```python
from build123d import *

# Parameters (mm, degrees)
F0_R     = 63.5
F1_DEPTH = 3.175


with BuildPart() as f1:
    # F0 (on Right) → F1 (new body)
    with BuildSketch(Plane.YZ):
        Circle(F0_R)
        with BuildLine():
            ThreePointArc((42.207203769, 42.207203769), (55.1463692956, 22.8423740779), (59.69, 0))
            ThreePointArc((59.69, 0), (56.4919386946, -19.2758128889), (47.240445216, -36.486112917))
            ThreePointArc((47.240445216, -36.486112917), (44.8152116738, -39.4270580012), (42.207203769, -42.207203769))
            ThreePointArc((42.207203769, -42.207203769), (22.8423740779, -55.1463692956), (0, -59.69))
            ThreePointArc((0, -59.69), (-19.2758128889, -56.4919386946), (-36.486112917, -47.240445216))
            ThreePointArc((-36.486112917, -47.240445216), (-39.4270580012, -44.8152116738), (-42.207203769, -42.207203769))
            ThreePointArc((-42.207203769, -42.207203769), (-55.1463692956, -22.8423740779), (-59.69, 0))
            ThreePointArc((-59.69, 0), (-56.4919386946, 19.2758128889), (-47.240445216, 36.486112917))
            ThreePointArc((-47.240445216, 36.486112917), (-44.8152116738, 39.4270580012), (-42.207203769, 42.207203769))
            ThreePointArc((-42.207203769, 42.207203769), (-22.8423740779, 55.1463692956), (0, 59.69))
            ThreePointArc((0, 59.69), (19.2758128889, 56.4919386946), (36.486112917, 47.240445216))
            ThreePointArc((36.486112917, 47.240445216), (39.4270580012, 44.8152116738), (42.207203769, 42.207203769))
        make_face(mode=Mode.SUBTRACT)
        with BuildLine():
            ThreePointArc((29.845, -29.845), (16.7276475457, -19.8525445451), (6.7351920908, -6.7351920908))
            ThreePointArc((6.7351920908, -6.7351920908), (3.6450596933, -8.7999525472), (0, -9.525))
            ThreePointArc((0, -9.525), (8.5432084009, -25.5734757664), (22.6607951031, -37.0292048969))
            Line((22.6607951031, -37.0292048969), (29.845, -29.845))
        make_face()
        with BuildLine():
            ThreePointArc((-6.7351920908, 6.7351920908), (-3.6450596933, 8.7999525472), (0, 9.525))
            ThreePointArc((0, 9.525), (-8.5432084009, 25.5734757664), (-22.6607951031, 37.0292048969))
            Line((-22.6607951031, 37.0292048969), (-29.845, 29.845))
            ThreePointArc((-29.845, 29.845), (-16.7276475457, 19.8525445451), (-6.7351920908, 6.7351920908))
        make_face()
        with BuildLine():
            ThreePointArc((6.7351920908, 6.7351920908), (8.7999525472, 3.6450596933), (9.525, 0))
            ThreePointArc((9.525, 0), (25.5734757664, 8.5432084009), (37.0292048969, 22.6607951031))
            Line((37.0292048969, 22.6607951031), (29.845, 29.845))
            ThreePointArc((29.845, 29.845), (19.8525445451, 16.7276475457), (6.7351920908, 6.7351920908))
        make_face()
        with BuildLine():
            ThreePointArc((-29.845, -29.845), (-19.8525445451, -16.7276475457), (-6.7351920908, -6.7351920908))
            ThreePointArc((-6.7351920908, -6.7351920908), (-8.7999525472, -3.6450596933), (-9.525, 0))
            ThreePointArc((-9.525, 0), (-25.5734757664, -8.5432084009), (-37.0292048969, -22.6607951031))
            Line((-37.0292048969, -22.6607951031), (-29.845, -29.845))
        make_face()
        with BuildLine():
            Line((-42.207203769, -42.207203769), (-29.845, -29.845))
            Line((-29.845, -29.845), (-37.0292048969, -22.6607951031))
            ThreePointArc((-37.0292048969, -22.6607951031), (-40.7112653305, -32.1444388979), (-42.207203769, -42.207203769))
        make_face()
        with BuildLine():
            Line((42.207203769, -42.207203769), (29.845, -29.845))
            Line((29.845, -29.845), (22.6607951031, -37.0292048969))
            ThreePointArc((22.6607951031, -37.0292048969), (32.1444388979, -40.7112653305), (42.207203769, -42.207203769))
        make_face()
        with BuildLine():
            Line((29.845, 29.845), (37.0292048969, 22.6607951031))
            ThreePointArc((37.0292048969, 22.6607951031), (40.7112653305, 32.1444388979), (42.207203769, 42.207203769))
            Line((42.207203769, 42.207203769), (29.845, 29.845))
        make_face()
        with BuildLine():
            Line((-29.845, 29.845), (-22.6607951031, 37.0292048969))
            ThreePointArc((-22.6607951031, 37.0292048969), (-32.1444388979, 40.7112653305), (-42.207203769, 42.207203769))
            Line((-42.207203769, 42.207203769), (-29.845, 29.845))
        make_face()
        with BuildLine():
            ThreePointArc((-36.486112917, -47.240445216), (-33.8273957569, -38.2900501722), (-29.845, -29.845))
            Line((-29.845, -29.845), (-42.207203769, -42.207203769))
            Line((-42.207203769, -42.207203769), (-36.486112917, -47.240445216))
        make_face()
        with BuildLine():
            ThreePointArc((47.240445216, -36.486112917), (38.2900501722, -33.8273957569), (29.845, -29.845))
            Line((29.845, -29.845), (42.207203769, -42.207203769))
            Line((42.207203769, -42.207203769), (47.240445216, -36.486112917))
        make_face()
        with BuildLine():
            ThreePointArc((36.486112917, 47.240445216), (33.8273957569, 38.2900501722), (29.845, 29.845))
            Line((29.845, 29.845), (42.207203769, 42.207203769))
            Line((42.207203769, 42.207203769), (36.486112917, 47.240445216))
        make_face()
        with BuildLine():
            ThreePointArc((-47.240445216, 36.486112917), (-38.2900501722, 33.8273957569), (-29.845, 29.845))
            Line((-29.845, 29.845), (-42.207203769, 42.207203769))
            Line((-42.207203769, 42.207203769), (-47.240445216, 36.486112917))
        make_face()
        with BuildLine():
            Line((9.525, 0), (1.651, 0))
            ThreePointArc((1.651, 0), (1.5253251082, -0.6318103468), (1.1674332957, -1.1674332957))
            Line((1.1674332957, -1.1674332957), (6.7351920908, -6.7351920908))
            ThreePointArc((6.7351920908, -6.7351920908), (8.7999525472, -3.6450596933), (9.525, 0))
        make_face()
        with BuildLine():
            ThreePointArc((-1.1674332957, 1.1674332957), (-0.6318103468, 1.5253251082), (0, 1.651))
            Line((0, 1.651), (0, 9.525))
            ThreePointArc((0, 9.525), (-3.6450596933, 8.7999525472), (-6.7351920908, 6.7351920908))
            Line((-6.7351920908, 6.7351920908), (-1.1674332957, 1.1674332957))
        make_face()
        with BuildLine():
            ThreePointArc((-1.651, 0), (-1.5253251082, 0.6318103468), (-1.1674332957, 1.1674332957))
            Line((-1.1674332957, 1.1674332957), (-6.7351920908, 6.7351920908))
            ThreePointArc((-6.7351920908, 6.7351920908), (-8.7999525472, 3.6450596933), (-9.525, 0))
            Line((-9.525, 0), (-1.651, 0))
        make_face()
        with BuildLine():
            Line((-6.7351920908, -6.7351920908), (-1.1674332957, -1.1674332957))
            ThreePointArc((-1.1674332957, -1.1674332957), (-1.5253251082, -0.6318103468), (-1.651, 0))
            Line((-1.651, 0), (-9.525, 0))
            ThreePointArc((-9.525, 0), (-8.7999525472, -3.6450596933), (-6.7351920908, -6.7351920908))
        make_face()
        with BuildLine():
            Line((0, -9.525), (0, -1.651))
            ThreePointArc((0, -1.651), (-0.6318103468, -1.5253251082), (-1.1674332957, -1.1674332957))
            Line((-1.1674332957, -1.1674332957), (-6.7351920908, -6.7351920908))
            ThreePointArc((-6.7351920908, -6.7351920908), (-3.6450596933, -8.7999525472), (0, -9.525))
        make_face()
        with BuildLine():
            Line((6.7351920908, -6.7351920908), (1.1674332957, -1.1674332957))
            ThreePointArc((1.1674332957, -1.1674332957), (0.6318103468, -1.5253251082), (0, -1.651))
            Line((0, -1.651), (0, -9.525))
            ThreePointArc((0, -9.525), (3.6450596933, -8.7999525472), (6.7351920908, -6.7351920908))
        make_face()
        with BuildLine():
            ThreePointArc((1.1674332957, 1.1674332957), (1.5253251082, 0.6318103468), (1.651, 0))
            Line((1.651, 0), (9.525, 0))
            Line((9.525, 0), (4.7625, 4.7625))
            Line((4.7625, 4.7625), (1.1674332957, 1.1674332957))
        make_face()
        with BuildLine():
            ThreePointArc((0, 1.651), (0.6318103468, 1.5253251082), (1.1674332957, 1.1674332957))
            Line((1.1674332957, 1.1674332957), (4.7625, 4.7625))
            Line((4.7625, 4.7625), (0, 9.525))
            Line((0, 9.525), (0, 1.651))
        make_face()
        with BuildLine():
            Line((4.7625, 4.7625), (9.525, 0))
            ThreePointArc((9.525, 0), (8.7999525472, 3.6450596933), (6.7351920908, 6.7351920908))
            Line((6.7351920908, 6.7351920908), (4.7625, 4.7625))
        make_face()
        with BuildLine():
            Line((0, 9.525), (4.7625, 4.7625))
            Line((4.7625, 4.7625), (6.7351920908, 6.7351920908))
            ThreePointArc((6.7351920908, 6.7351920908), (3.6450596933, 8.7999525472), (0, 9.525))
        make_face()
        with BuildLine():
            Line((-47.240445216, 36.486112917), (-42.207203769, 42.207203769))
            ThreePointArc((-42.207203769, 42.207203769), (-44.8152116738, 39.4270580012), (-47.240445216, 36.486112917))
        make_face()
        with BuildLine():
            Line((-36.486112917, -47.240445216), (-42.207203769, -42.207203769))
            ThreePointArc((-42.207203769, -42.207203769), (-39.4270580012, -44.8152116738), (-36.486112917, -47.240445216))
        make_face()
        with BuildLine():
            Line((47.240445216, -36.486112917), (42.207203769, -42.207203769))
            ThreePointArc((42.207203769, -42.207203769), (44.8152116738, -39.4270580012), (47.240445216, -36.486112917))
        make_face()
        with BuildLine():
            Line((36.486112917, 47.240445216), (42.207203769, 42.207203769))
            ThreePointArc((42.207203769, 42.207203769), (39.4270580012, 44.8152116738), (36.486112917, 47.240445216))
        make_face()
    extrude(amount=F1_DEPTH)


solid = f1.part
```
Verification items for the finished model (mm, model axes). A direction names the side the tool comes from. Give positions to 0.01 mm unless a question says otherwise; leave off trailing zeros. Loops run counter-clockwise (first coordinate to the right, second up) from the corner with the lowest first, then second, coordinate; pieces in that order, holes last. Notation, with made-up numbers: M -39.5,33.5 L -11.5,33.5 A21 cw -11.5,72.5 Z; hole C 36.5,-32.75 d9. An arc over 180 degrees is marked long. Return JSON: item names as keys, results as strings.
1) Material ranges on L1, parallel to Z at x = 0.95, y = -18; L2, parallel to Z at x = 2.3, y = -12; L3, parallel to Y at x = 0.9, z = 38.5, recorded low to high. Write a range as [from, to].
Findings:
{"L1": "z = [-60.9, -56.91], [-14.95, -3.48], [21.09, 34.23], [56.91, 60.9]", "L2": "z = [-62.36, -58.47], [-10.09, -0.81], [14.54, 29.32], [58.47, 62.36]", "L3": "y = [-50.5, -25.75], [33.91, 41.92], [45.61, 50.5]"}
2) Gauge pin test, flat ends, axial feed: P1, Ø1.5, axis at x = 1.5, y = -24, coming from the -Z side; P2, Ø1, axis at x = 1, y = -45, coming from the -Z side; P3, Ø8, axis at y = -2, z = 23, coming from the -X side; P4, Ø1.5, axis at x = 2, z = -42, coming from the -Y side. Record the tip position at first contact, or that the pin passes through.
Findings:
{"P1": "stops at z = -59.09", "P2": "stops at z = -45.3", "P3": "stops at x = 0", "P4": "stops at y = -48.28"}
3) Tool access check on faces 4 (the cylindrical face through (1.57, -8.78, 3.69)), 5 (the flat face through (0, 0, 5)). Record the directions out of +Z, -Z, +X, -X, +Y, -Y that give a thin tool (end or side, any length) a straight path to the whole face; none if there is none.
Findings:
{"face 4": "+X, -X", "face 5": "+Z, -Z, -X, +Y, -Y"}
4) Section check A-A, the plane y = -28. Enter the section's corners in (x, z) (3 decimals), and give its area (3 significant figures).
Findings:
{"outline": "M 0,-56.993 L 3.175,-56.993 L 3.175,-52.715 L 0,-52.715 Z; M 0,-26.805 L 3.175,-26.805 L 3.175,-10.691 L 0,-10.691 Z; M 0,28.754 L 3.175,28.754 L 3.175,39.4 L 0,39.4 Z; M 0,52.715 L 3.175,52.715 L 3.175,56.993 L 0,56.993 Z", "area": "112 mm2"}
5) Mould release check, pull along Z, two halves, no side actions. Record for faces 1 (the cylindrical face through (1.57, -13.77, -61.99)), 2 (the cylindrical face through (1.57, -3.69, -8.78)), 3 (the flat face through (3.175, 0, 5)): released by +Z, released by -Z, zero draft, split by the parting line, or undercut.
Findings:
{"face 1": "split by the parting line", "face 2": "undercut", "face 3": "zero draft"}
6) Section check B-B, the plane x = 2.25. Enter the section's corners in (y, z) (3 decimals), and give its area (3 significant figures).
Findings:
{"outline": "C 0,0 d127; hole M -47.24,36.486 A59.69 ccw -42.207,-42.207 A45.764 cw -9.525,0 A9.525 cw -6.735,6.735 A61.529 ccw Z; hole M -42.207,42.207 A45.764 cw 0,9.525 A9.525 cw 6.735,6.735 A61.529 ccw 36.486,47.24 A59.69 ccw Z; hole M -36.486,-47.24 A59.69 ccw 42.207,-42.207 A45.764 cw 0,-9.525 A9.525 cw -6.735,-6.735 A61.529 ccw Z; hole C 0,0 d3.302; hole M 6.735,-6.735 A61.529 ccw 47.24,-36.486 A59.69 ccw 42.207,42.207 A45.764 cw 9.525,0 A9.525 cw Z", "area": "3,700 mm2"}
